Could you check a few things on this model? Use its own coordinates, in mm. Coordinates: 2 decimals unless noted, no trailing zeros. Order: outer loops, then holes, each group sorted by start corner. A loop starts at its lowest first (then second) coordinate and runs counter-clockwise, first axis right, second up. Notation, with made-up numbers: (73.25, 76.5) - (131.25, 76.5) arc R25 cw to (131.25, 111.5) - close; hole circle Ø9 at (-22.5, 19). An arc over 180 degrees is marked (long way). Answer as a JSON object with one key per item and string values. Group by question number.
(1) Imagine slicing it at C-C, the plane z = 1.9. Write out the boundary of the cut face in (x, y), and give its area (3 significant figures).
(2) Imagine slicing it at A-A, the plane x = 0. Write out the boundary of the cut face in (y, z) (3 decimals), and give its area (3 significant figures).
(3) Will this pin go through, and if not, where does the flat tip stop? P1, Ø3, axis at x = 26.5, y = 26.5, coming from the -Z side.
(4) Imagine slicing it at B-B, the plane y = 25.4. Write out the boundary of the cut face in (x, z) (3 decimals).
(5) Imagine slicing it at D-D, the plane x = -17. Write out the boundary of the cut face in (y, z) (3 decimals).
(6) We'd pull the mould along X, two halves only. Please class faces 1 (the flat face through (-38.1, -1, 2)), 2 (the flat face through (-1, 9, 3.175)), 3 (the cylindrical face through (19.78, 22.1, 1.57)): pulls with the +X half, pulls with the -X half, needs draft (parallel to the pull), parting line crosses it, or undercut.
(7) Please list where these lines run through material, in increasing order: probe 1 along Y at (x, z) = (0, 1); probe 2 along Y at (x, z) = (-19.05, 1.55); probe 3 along X at (y, z) = (-16.5, 2.45).
from build123d import *

# Parameters (mm, degrees)
SKETCH1_W               = 76.2
SKETCH1_H               = 76.2
BOSS_EXTRUDE1_DEPTH     = 3.175
F_1_4_CLEARANCE_HOLE1_D = 6.7564
CUT_EXTRUDE1_DEPTH      = 54.975
CUT_EXTRUDE1_DEPTH_BACK = 54.975
SKETCH4_R               = 14.77


with BuildPart() as part:
    # Sketch1 → Boss-Extrude1 (new body)
    with BuildSketch(Plane.XY):
        Rectangle(SKETCH1_W, SKETCH1_H)
    extrude(amount=BOSS_EXTRUDE1_DEPTH)

    # 1/4 Clearance Hole1 (through all)
    with Locations(Plane.XY.offset(3.175)):
        with Locations((19.05, 25.4), (-19.05, 25.4)):
            Hole(F_1_4_CLEARANCE_HOLE1_D / 2)

    # Sketch4 → Cut-Extrude1 (cut, two sides: drawn at the far end of the back side and taken through both)
    with BuildSketch(Plane.XY.offset(3.175).offset(-CUT_EXTRUDE1_DEPTH_BACK)):
        with Locations((0, -12.552196451)):
            Circle(SKETCH4_R)
    extrude(amount=CUT_EXTRUDE1_DEPTH + CUT_EXTRUDE1_DEPTH_BACK, mode=Mode.SUBTRACT)


solid = part.part
Result set:
{
 "1": {"outline": "(-38.1, -38.1) - (38.1, -38.1) - (38.1, 38.1) - (-38.1, 38.1) - close; hole circle Ø6.76 at (-19.05, 25.4); hole circle Ø29.54 at (0, -12.55); hole circle Ø6.76 at (19.05, 25.4)", "area": "5,050 mm^2"},
 "2": {"outline": "(-38.1, 0) - (-27.322, 0) - (-27.322, 3.175) - (-38.1, 3.175) - close; (2.218, 0) - (38.1, 0) - (38.1, 3.175) - (2.218, 3.175) - close", "area": "148 mm^2"},
 "3": {"P1": "stops at z = 0"},
 "4": {"outline": "(-38.1, 0) - (-22.428, 0) - (-22.428, 3.175) - (-38.1, 3.175) - close; (-15.672, 0) - (15.672, 0) - (15.672, 3.175) - (-15.672, 3.175) - close; (22.428, 0) - (38.1, 0) - (38.1, 3.175) - (22.428, 3.175) - close"},
 "5": {"outline": "(-38.1, 0) - (22.715, 0) - (22.715, 3.175) - (-38.1, 3.175) - close; (28.085, 0) - (38.1, 0) - (38.1, 3.175) - (28.085, 3.175) - close"},
 "6": {"face 1": "pulls with the -X half", "face 2": "needs draft", "face 3": "undercut"},
 "7": {"probe 1": "y = -38.1 to -27.32, 2.22 to 38.1", "probe 2": "y = -38.1 to 22.02, 28.78 to 38.1", "probe 3": "x = -38.1 to -14.23, 14.23 to 38.1"}
}
